The listing builds one solid part. Answer for the finished solid, in the listing's coordinates (mm). A direction names the side the tool comes from. Coordinates: 2 decimals unless noted, no trailing zeros. Write each loop counter-clockwise with the first axis right and the second up, starting at its lowest first coordinate (ties: lowest second). Pieces come first, ordered by that corner, then holes.
from build123d import *

# Parameters (mm, degrees)
F0_R     = 9.525
F1_DEPTH = 12.7
F3_DEPTH = 6.35
F4_W     = 25.4
F4_H     = 25.4
F5_DEPTH = 12.7
F7_DEPTH = 34.926
F8_R     = 6.35
F9_DEPTH = 25.401


with BuildPart() as f1:
    # F0 (on Front) → F1 (new body, symmetric)
    with BuildSketch(Plane.XZ):
        Circle(F0_R)
    extrude(amount=F1_DEPTH, both=True)

    # F2 (on Front) → F3 (join, symmetric)
    with BuildSketch(Plane.XZ):
        with BuildLine():
            ThreePointArc((0, -9.581195), (-9.525, -0.056195), (0, 9.468805))
            Line((0, 9.468805), (-12.7, 9.468805))
            Line((-12.7, 9.468805), (-12.7, -9.581195))
            Line((-12.7, -9.581195), (0, -9.581195))
        make_face()
    extrude(amount=F3_DEPTH, both=True)

    # F4 (on face) → F5 (join)
    with BuildSketch(Plane(origin=(-12.7, 0, 0), x_dir=(0, -1, 0), z_dir=(-1, 0, 0))):
        with Locations((0, 3.118805)):
            Rectangle(F4_W, F4_H)
    extrude(amount=F5_DEPTH)

    # F6 (on face) → F7 (cut, through all)
    with BuildSketch(Plane(origin=(-25.4, 0, 0), x_dir=(0, -1, 0), z_dir=(-1, 0, 0))):
        Polygon((-6.35, 15.818805), (-12.7, 15.818805), (-12.7, 9.468805), align=None)
        Polygon((12.7, 9.468805), (12.7, 15.818805), (6.35, 15.818805), align=None)
    extrude(amount=-F7_DEPTH, mode=Mode.SUBTRACT)

    # F8 (on face) → F9 (cut, through all)
    with BuildSketch(Plane.XZ.offset(12.7)):
        Circle(F8_R)
    extrude(amount=-F9_DEPTH, mode=Mode.SUBTRACT)


solid = f1.part
Q1. Determine the mould class of faces 1 (the face through (-19.14, 9.57, 12.6)), 2 (the face through (-1.38, -0.18, -6.2)), 3 (the face through (-19, 12.7, 0)), 4 (the face through (-15, 0, -9.581)) for opening direction Z: released by +Z, released by -Z, zero draft, split by the parting line, or undercut.
Answers below:
face 1: released by +Z
face 2: undercut
face 3: zero draft
face 4: released by -Z
Q2. The part is cut by section C-C, the plane x = -23. Write down the section's boundary in (y, z), then the cut area to 3 significant figures.
Answers below:
outline: (-12.7, -9.58) - (12.7, -9.58) - (12.7, 9.47) - (6.35, 15.82) - (-6.35, 15.82) - (-12.7, 9.47) - close
area: 605 mm2
Q3. Which of the six approach directions +Z, -Z, +X, -X, +Y, -Y give full straight-line access (tool end or side, diameter ignored) to faces 5 (the face through (-11, -6.35, 0)), 6 (the face through (-7, 0, 9.469)), 7 (the face through (-12.7, 0, 12)), 8 (the face through (-11, 6.35, 0))?
Answers below:
face 5: -Y
face 6: +Z, +Y, -Y
face 7: +Z
face 8: +Y
Q4. Find the intervals of material crossed by probe 1 along X at (y, z) = (-8.5, 1.25); probe 2 along X at (y, z) = (11.5, 0.5); probe 3 along X at (y, z) = (-9, 8.25), in increasing order.
Answers below:
probe 1: x = -25.4 to -12.7, -9.44 to -6.23, 6.23 to 9.44
probe 2: x = -25.4 to -12.7, -9.51 to -6.33, 6.33 to 9.51
probe 3: x = -25.4 to -12.7, -4.76 to 4.76
Q5. Given pin 1 (6 mm diameter, centred on x = -8.5, y = -2, fed in from +Z); pin 2 (2 mm diameter, centred on y = -3, z = -1.5, fed in from +X); pin 3 (1.5 mm diameter, centred on x = -10, z = 11.5, fed in from -Y), each flat-ended and moving along its own axis, determine where each tip first touches the part or whether it passes through.
Answers below:
pin 1: stops at z = 9.47
pin 2: stops at x = 9.51
pin 3: passes through
Q6. The part is cut by section D-D, the plane y = -2.25. Write down the section's boundary in (x, z) (3 decimals).
Answers below:
outline: (-25.4, -9.581) - (0, -9.581) arc R9.525 cw to (-9.525, -0.028) arc R9.525 ccw (long way) to (-1.033, 9.469) - (-12.7, 9.469) - (-12.7, 15.819) - (-25.4, 15.819) - close; hole circle Ø12.7 at (0, 0)
Q7. The part is cut by section B-B, the plane y = -7.5. Write down the section's boundary in (x, z) (3 decimals), then the cut area to 3 significant figures.
Answers below:
outline: (-25.4, -9.581) - (-12.7, -9.581) - (-12.7, 14.669) - (-25.4, 14.669) - close; circle Ø19.05 at (0, 0); hole circle Ø12.7 at (0, 0)
area: 466 mm2
Q8. The part is cut by section A-A, the plane z = -0.5. Write down the section's boundary in (x, y).
Answers below:
outline: (-25.4, -12.7) - (-12.7, -12.7) - (-12.7, -6.35) - (-9.51, -6.35) - (-9.51, 6.35) - (-12.7, 6.35) - (-12.7, 12.7) - (-25.4, 12.7) - close; (-9.51, -12.7) - (-6.33, -12.7) - (-6.33, 12.7) - (-9.51, 12.7) - close; (6.33, -12.7) - (9.51, -12.7) - (9.51, 12.7) - (6.33, 12.7) - close
